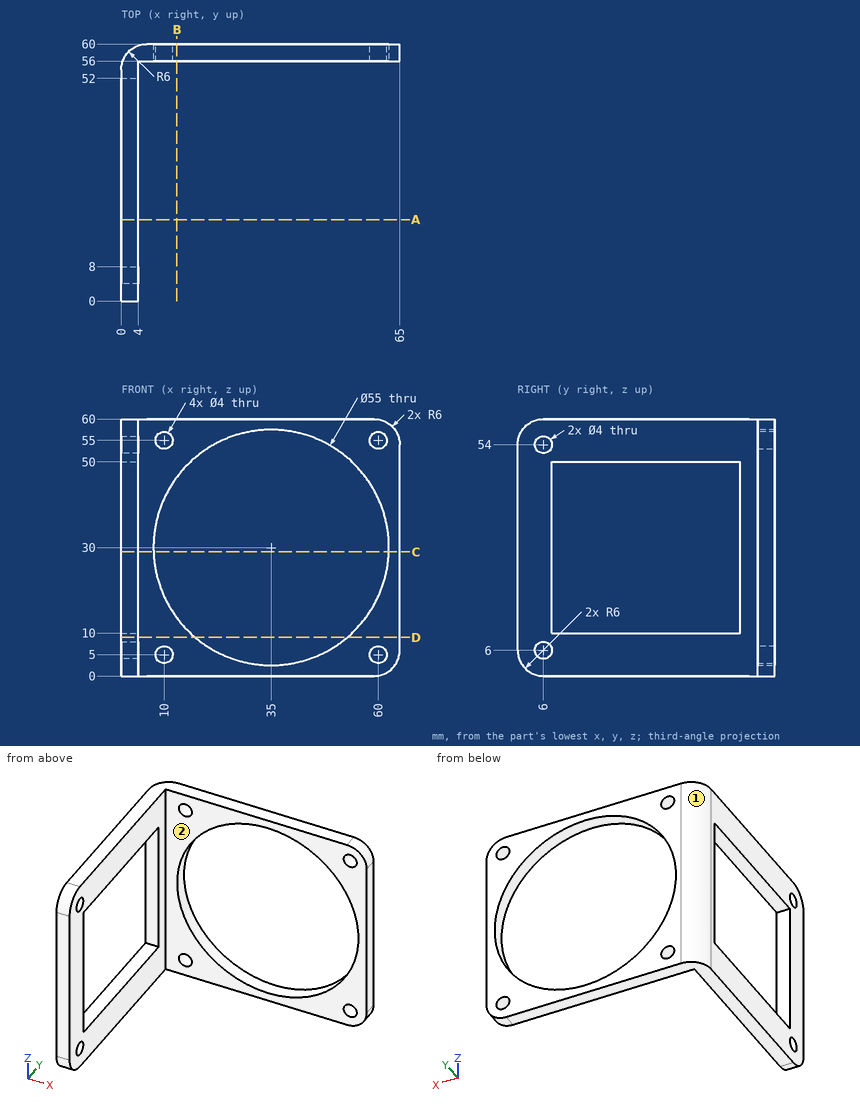
Geometry check sheet. Reference: drawing and pictorial views, mm from the part's lowest x, y, z. A direction names the side the tool comes from. Coordinates: 2 decimals unless noted, no trailing zeros. Loops run counter-clockwise (first coordinate to the right, second up) from the corner with the lowest first, then second, coordinate; pieces in that order, holes last.
1) Sectioned sample at B-B (x = 13). Record the boundary of the cut face in (y, z), and give its area (3 significant figures).
2) Gauge pin test, flat ends, axial feed: pin 1 (5 mm diameter, centred on y = 6, z = 54, fed in from +X); pin 2 (5 mm diameter, centred on x = 60, z = 5, fed in from -Y); pin 3 (4.5 mm diameter, centred on x = 2.5, z = 40, fed in from +Y); pin 4 (2 mm diameter, centred on x = 1.5, z = 32.5, fed in from -Y). Record the tip position at first contact, or that the pin passes through.
3) Material ranges on probe 1 along Y at (x, z) = (60.5, 45.5); probe 2 along X at (y, z) = (57, 55); probe 3 along X at (y, z) = (3.5, 25), recorded low to high.
4) Sectioned sample at A-A (y = 19). Record the boundary of the cut face in (x, z).
5) Sectioned sample at D-D (z = 9). Record the boundary of the cut face in (x, y), and give its area (3 significant figures).
6) Sectioned sample at C-C (z = 29). Record the boundary of the cut face in (x, y).
7) Access from +Z, -Z, +X, -X, +Y, -Y to the whole of each face (thin tool, end or side, straight path). Record for the marked faces 1 and 2.
Check sheet entries:
1. outline: (56, 0) - (60, 0) - (60, 13.5) - (56, 13.5) - close; (56, 46.5) - (60, 46.5) - (60, 60) - (56, 60) - close
1. area: 108 mm2
2. pin 1: stops at x = 4
2. pin 2: stops at y = 56
2. pin 3: stops at y = 59.87
2. pin 4: stops at y = 0
3. probe 1: y = 56 to 60
3. probe 2: x = 0.8 to 8, 12 to 23.54, 46.46 to 58, 62 to 64.92
3. probe 3: x = 0 to 4
4. outline: (0, 0) - (4, 0) - (4, 10) - (0, 10) - close; (0, 50) - (4, 50) - (4, 60) - (0, 60) - close
5. outline: (0, 0) - (4, 0) - (4, 56) - (17.24, 56) - (17.24, 60) - (6, 60) arc R6 ccw to (0, 54) - close; (52.76, 56) - (65, 56) - (65, 60) - (52.76, 60) - close
5. area: 334 mm2
6. outline: (0, 0) - (4, 0) - (4, 8) - (0, 8) - close; (0, 52) - (4, 52) - (4, 56) - (7.52, 56) - (7.52, 60) - (6, 60) arc R6 ccw to (0, 54) - close; (62.48, 56) - (65, 56) - (65, 60) - (62.48, 60) - close
7. face 1: +Z, -Z, -X, +Y
7. face 2: +Z, -Z, +X, -Y
